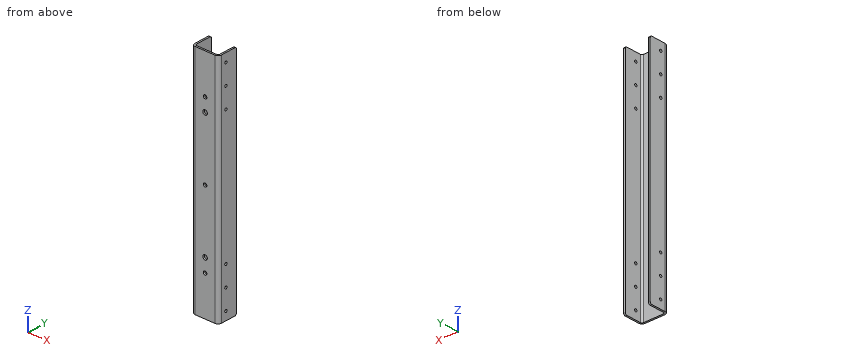
from build123d import *

# Parameters (mm, degrees)
BASE_FLANGE1_DEPTH = 434.975
SKETCH8_R          = 4.3688
SKETCH8_R_2        = 3.3782
CUT_EXTRUDE2_DEPTH = 440.585601021
SKETCH9_R          = 2.4257
CUT_EXTRUDE3_DEPTH = 440.585601021
FILLET1_R          = 3.175


# Sheet-metal steps are written as plain solids
with BuildPart() as part:
    # Sketch1 → Base-Flange1 (new body)
    with BuildSketch(Plane.XY):
        with BuildLine():
            Line((50.8, 38.1), (50.8, 6.35))
            ThreePointArc((50.8, 6.35), (48.940128061, 1.859871939), (44.45, 0))
            Line((44.45, 0), (6.35, 0))
            ThreePointArc((6.35, 0), (1.859871939, 1.859871939), (0, 6.35))
            Line((0, 6.35), (0, 38.1))
            Line((0, 38.1), (3.175, 38.1))
            Line((3.175, 38.1), (3.175, 6.35))
            ThreePointArc((3.175, 6.35), (4.10493597, 4.10493597), (6.35, 3.175))
            Line((6.35, 3.175), (44.45, 3.175))
            ThreePointArc((44.45, 3.175), (46.69506403, 4.10493597), (47.625, 6.35))
            Line((47.625, 6.35), (47.625, 38.1))
            Line((47.625, 38.1), (50.8, 38.1))
        make_face()
    extrude(amount=BASE_FLANGE1_DEPTH)

    # Sketch8 → Cut-Extrude2 (cut, through all)
    with BuildSketch(Plane.XZ):
        with Locations(Location((25.4, 100.0125, 0), (0, 0, 270))):
            Circle(SKETCH8_R)
        with Locations(Location((25.4, 334.9625, 0), (0, 0, 270))):
            Circle(SKETCH8_R)
        with Locations(Location((25.4, 217.4875, 0), (0, 0, 270))):
            Circle(SKETCH8_R_2)
        with Locations(Location((25.4, 74.6125, 0), (0, 0, 270))):
            Circle(SKETCH8_R_2)
        with Locations(Location((25.4, 360.3625, 0), (0, 0, 270))):
            Circle(SKETCH8_R_2)
    extrude(amount=-CUT_EXTRUDE2_DEPTH, mode=Mode.SUBTRACT)

    # Sketch9 → Cut-Extrude3 (cut, through all)
    with BuildSketch(Plane(origin=(50.8, 0, 0), x_dir=(0, 0, -1), z_dir=(1, 0, 0))):
        with Locations((-419.1, 15.875)):
            Circle(SKETCH9_R)
        with Locations((-381, 15.875)):
            Circle(SKETCH9_R)
        with Locations((-342.9, 15.875)):
            Circle(SKETCH9_R)
        with Locations((-92.075, 15.875)):
            Circle(SKETCH9_R)
        with Locations((-53.975, 15.875)):
            Circle(SKETCH9_R)
        with Locations((-15.875, 15.875)):
            Circle(SKETCH9_R)
    extrude(amount=-CUT_EXTRUDE3_DEPTH, mode=Mode.SUBTRACT)

    # Fillet1
    fillet1_edges = [part.edges().sort_by_distance(p)[0] for p in [
        (1.5875, 38.1, 0),
        (49.2125, 38.1, 0),
        (1.5875, 38.1, 434.975),
        (49.2125, 38.1, 434.975),
    ]]
    fillet(fillet1_edges, radius=FILLET1_R)


solid = part.part
Verification items for the finished model (mm, model axes). Give positions to 0.01 mm unless a question says otherwise; leave off trailing zeros. Write each loop counter-clockwise with the first axis right and the second up, starting at its lowest first coordinate (ties: lowest second). Pieces come first, ordered by that corner, then holes.
(1) Cross-section at A-A (y = 26). Enter the section's corners in (x, z) (3 decimals).
(2) Cross-section at B-B (z = 205.5). Enter the section's corners in (x, y) (3 decimals).
(3) Material ranges on line 1 (Z direction, x = 25, y = 2) (3 decimals); line 2 (X direction, y = 31, z = 150.5) (3 decimals); line 3 (Y direction, x = 21, z = 41.5) (3 decimals), recorded low to high.
(4) Gauge pin test, flat end, axial feed: pin 1 (3 mm diameter, centred on x = 28.5, z = 252, fed in from +Y) (3 decimals). Record the tip position at first contact, or that the pin passes through.
Worked out:
1. outline: (0, 0) - (3.175, 0) - (3.175, 434.975) - (0, 434.975) - close; (47.625, 0) - (50.8, 0) - (50.8, 434.975) - (47.625, 434.975) - close
2. outline: (0, 6.35) arc R6.35 ccw to (6.35, 0) - (44.45, 0) arc R6.35 ccw to (50.8, 6.35) - (50.8, 38.1) - (47.625, 38.1) - (47.625, 6.35) arc R3.175 cw to (44.45, 3.175) - (6.35, 3.175) arc R3.175 cw to (3.175, 6.35) - (3.175, 38.1) - (0, 38.1) - close
3. line 1: z = 0 to 71.258, 77.967 to 95.662, 104.363 to 214.133, 220.842 to 330.612, 339.313 to 357.008, 363.717 to 434.975
3. line 2: x = 0 to 3.175, 47.625 to 50.8
3. line 3: y = 0 to 3.175
4. pin 1: stops at y = 3.175
